Geometry check sheet. Reference: the model listing, model coordinates, mm. A direction names the side the tool comes from. Coordinates: 2 decimals unless noted, no trailing zeros. Order: outer loops, then holes, each group sorted by start corner. A loop starts at its lowest first (then second) coordinate and runs counter-clockwise, first axis right, second up. Notation, with made-up numbers: (30.25, 10.5) - (38.25, 10.5) arc R24 ccw to (38.25, 29.5) - close; hole circle Ø8 at (22.5, 55.5). An arc over 180 degrees is marked (long way). One line per item, written item: value. Start each with the question number.
Autodesk Inventor part; units mm, degrees
ref_plane "YZ Plane" through (0, 0, 0) normal (1, 0, 0) x (0, 1, 0)
ref_plane "XZ Plane" through (0, 0, 0) normal (0, 1, 0) x (-1, 0, 0)
ref_plane "XY Plane" through (0, 0, 0) normal (0, 0, 1) x (1, 0, 0)
sketch "スケッチ1" plane through (0, 0, 0) normal (1, 0, 0) x (0, 1, 0)
  line L0 (-670, 192.9198) -> (-670, 500)
  line L1 (-670, 500) -> (-350, 650)
  line L2 (-350, 650) -> (-90, 650)
  line L3 (0, 250) -> (0, 0)
  line L4 (-124.5856, 512.0252) -> (-145.1979, 512.0252)
  line L5 (-145.1979, 512.0252) -> (0, 250)
  line L6 (-90, 650) -> (-124.5856, 512.0252)
  line L7 (-249.1712, 52.2397) -> (-510, 192.9198)
  line L8 (-510, 192.9198) -> (-670, 192.9198)
  line L9 (0, 0) -> (-249.1712, 52.2397)
  dimension "d2" = 150
  dimension "d3" = 320
  dimension "d4" = 250
  dimension "d5" = 670
  dimension "d79" = 260
extrude "押し出し1" add sketch "スケッチ1" along normal blind 5
sketch "スケッチ8" plane through (5, 0, 0) normal (1, 0, 0) x (0, 0, -1)
  circle A0 centre (-570, -250) radius 7.5
  circle A1 centre (-288.2903, -224.7089) radius 7.5
  line L0 (0, 0) -> (-250, 0)
  line L1 (-570, -250) -> (-290.3837, -264.6541)
  line L2 (-290.3837, -264.6541) -> (-288.2903, -224.7089)
  line L3 (0, -804) -> (0, 134)
  dimension "d65" = 15
  dimension "d66" = 15
  dimension "d77" = 250
  dimension "d88" = 40
  dimension "d89" = 280
  dimension "d90" = 3
  dimension "d91" = 570
extrude "押し出し8" cut sketch "スケッチ8" against normal through all
sketch "スケッチ12" plane through (5, 0, 0) normal (1, 0, 0) x (0, 0, -1)
  circle A0 centre (-200, -95) radius 6.6799
  point P0 (0, 0)
  dimension "d84" = 200
  dimension "d85" = 95
extrude "押し出し11" cut sketch "スケッチ12" against normal through all
sketch "スケッチ13" plane through (5, 0, 0) normal (1, 0, 0) x (0, 0, -1)
  line L0 (0, -804) -> (0, 134)
  line L1 (130, 0) -> (-780, 0)
  line L2 (-80, 0) -> (-121.7476, -89.528)
  line L3 (-121.7476, -89.528) -> (-1.0516, -5.0157)
  line L4 (-52.2397, -249.1712) -> (0, 0)
  dimension "d95" = 80
  dimension "d96" = 115
  dimension "d97" = 30
extrude "押し出し12" cut sketch "スケッチ13" against normal through all
fillet "フィレット2" radius 3 6 edges at (2.5, -89.528, 121.7476) (2.5, -5.0157, 1.0516) (2.5, 0, 80) (2.5, -145.1979, 512.0252) (2.5, -124.5856, 512.0252) (2.5, -90, 650)
sketch "スケッチ14" plane through (5, 0, 0) normal (1, 0, 0) x (0, 0, -1)
  line L0 (-117.0159, -79.3808) -> (-81.9901, -4.2679)
  line L1 (-52.2397, -249.1712) -> (-2.608, -12.4393)
  line L2 (-7.2648, -9.3663) -> (-112.5762, -83.1061)
  line L3 (-81.9901, -4.2679) -> (-147.7654, -145.3235)
  line L4 (-147.7654, -145.3235) -> (-18.9575, -90.4227)
  line L5 (-52.2397, -249.1712) -> (-2.608, -12.4393)
  line L6 (-18.9575, -90.4227) -> (-2.608, -12.4393)
  line L7 (-2.608, -12.4393) -> (0, 0)
  line L8 (0, 0) -> (-81.9901, -4.2679)
extrude "押し出し13" cut sketch "スケッチ14" against normal through all
fillet "フィレット3" radius 2 2 edges at (2.5, -145.3235, 147.7654) (2.5, -90.4227, 18.9575)
properties part number "end_plate" material "木材 (オーク)"
Q1. Gauge pin test, flat ends, axial feed: P1, Ø3, axis at x = 4, z = 367, coming from the +Y side; P2, Ø3, axis at x = 1, y = -373, coming from the -Z side; P3, Ø3, axis at x = 3, y = -582.5, coming from the -Z side. Record the tip position at first contact, or that the pin passes through.
Q2. Set-up check for faces 1 (the flat face through (2.465, -377.76, 121.595)), 2 (the flat face through (2.54, -117.96, 83.57)), 3 (the flat face through (2.465, -107.244, 581.207)): record each of +Z, -Z, +X, -X, +Y, -Y from which the full face is reachable in a straight line by a thin tool's end or side.
Q3. Release check for a two-part mould opening along Z. For faces 4 (the flat face through (0, -340, 339)), 5 (the flat face through (2.465, -170.589, 35.765)), 6 (the flat face through (2.465, -72.364, 380.589)), 7 (the flat face through (2.46, -512.24, 573.95)) record: released by +Z, released by -Z, zero draft, split by the parting line, or undercut.
Q4. Cross-section at B-B, the plane x = 1.15. Enter the section's corners in (y, z).
Q5. Cross-section at A-A, the plane z = 570. Enter the section's corners in (x, y), and give its area (3 significant figures).
Q6. Material ranges on probe 1 along Y at (x, z) = (2.05, 200); probe 2 along Y at (x, z) = (2.3, 111.5); probe 3 along Z at (x, y) = (3.7, -225), recorded low to high.
Q7. Cross-section at C-C, the plane y = -62. Enter the section's corners in (x, z), and give its area (3 significant figures).
Q8. Cross-section at D-D, the plane z = 129. Enter the section's corners in (x, y), and give its area (3 significant figures).
Check result:
1. P1: stops at y = -64
1. P2: stops at z = 118.22
1. P3: stops at z = 192.92
2. face 1: -Z, +X, -X, -Y
2. face 2: +X, -X
2. face 3: +X, -X, +Y
3. face 4: zero draft
3. face 5: released by -Z
3. face 6: undercut
3. face 7: released by +Z
4. outline: (-670, 192.92) - (-510, 192.92) - (-249.17, 52.24) - (-94.18, 19.74) arc R2 ccw to (-91.93, 22.49) - (-143.28, 142.96) arc R2 cw to (-140.59, 145.56) - (-79.38, 117.02) - (-4.27, 81.99) arc R3 ccw to (0, 84.71) - (0, 250) - (-142.73, 507.57) arc R3 cw to (-140.11, 512.03) - (-126.93, 512.03) arc R3 ccw to (-124.02, 514.3) - (-90.93, 646.27) arc R3 ccw to (-93.84, 650) - (-350, 650) - (-670, 500) - close; hole circle Ø15 at (-250, 570); hole circle Ø15 at (-224.71, 288.29); hole circle Ø13.36 at (-95, 200)
5. outline: (0, -520.67) - (5, -520.67) - (5, -257.5) - (0, -257.5) - close; (0, -242.5) - (5, -242.5) - (5, -110.05) - (0, -110.05) - close
5. area: 1,980 mm2
6. probe 1: y = -670 to -101.68, -88.32 to 0
6. probe 2: y = -359.04 to -129.87, -67.55 to 0
6. probe 3: z = 47.17 to 280.8, 295.78 to 650
7. outline: (0, 108.91) - (5, 108.91) - (5, 361.89) - (0, 361.89) - close
7. area: 1,260 mm2
8. outline: (0, -391.49) - (5, -391.49) - (5, -137.33) - (0, -137.33) - close; (0, -105.08) - (5, -105.08) - (5, 0) - (0, 0) - close
8. area: 1,800 mm2
